from build123d import *

# Parameters (mm, degrees)
F0_W     = 266.7
F0_H     = 152.4
F1_DEPTH = 50.8
F2_R     = 19.05
F3_DEPTH = 50.801
F4_R     = 19.05
F5_DEPTH = 50.801
F6_R     = 6.35


with BuildPart() as f1:
    # F0 (on Front) → F1 (new body)
    with BuildSketch(Plane.XZ):
        Rectangle(F0_W, F0_H)
    extrude(amount=F1_DEPTH)

    # F2 (on Front) → F3 (cut, through all)
    with BuildSketch(Plane.XZ):
        Circle(F2_R)
    extrude(amount=F3_DEPTH, mode=Mode.SUBTRACT)

    # F4 (on Front) → F5 (cut, through all)
    with BuildSketch(Plane.XZ):
        with Locations((-63.5, 0)):
            Circle(F4_R)
        with BuildLine():
            ThreePointArc((82.55, 0), (63.5, 19.05), (44.45, 0))
            ThreePointArc((44.45, 0), (63.5, -19.05), (82.55, 0))
        make_face()
    extrude(amount=F5_DEPTH, mode=Mode.SUBTRACT)

    # F6
    f6_edges = [f1.edges().sort_by_distance(p)[0] for p in [
        (-133.35, -50.8, 0),
        (0, -50.8, -76.2),
        (0, -50.8, 76.2),
        (133.35, -50.8, 0),
        (-133.35, -25.4, -76.2),
        (0, 0, -76.2),
        (-133.35, 0, 0),
        (133.35, -25.4, -76.2),
        (133.35, 0, 0),
        (0, 0, 76.2),
    ]]
    fillet(f6_edges, radius=F6_R)


solid = f1.part
Input: part model. Units: mm. Frame: model coordinates. Coordinates: 2 decimals unless noted, no trailing zeros. Loops run counter-clockwise (first coordinate to the right, second up) from the corner with the lowest first, then second, coordinate; pieces in that order, holes last. Notation, with made-up numbers: (-10, 48) -> (41, 48) arc R4 ccw to (41, 55) -> close; hole circle Ø2 at (-28.5, 51.5). An arc over 180 degrees is marked (long way). Write item = value, one per line. Start each with the question number.
Item 1: Cut plane C-C, the plane y = -11. Return loops of the section in (x, z), plus the area to 3 significant figures.
Item 2: Cut plane A-A, the plane x = 63.5. Return loops of the section in (y, z).
Item 3: Material intervals for line 1 (X direction, y = -3.5, z = 3); line 2 (X direction, y = -46.5, z = 1); line 3 (Z direction, x = 0, y = -32), sorted ascending.
Item 4: Cut plane D-D, the plane x = -53.5. Return loops of the section in (y, z), plus the area to 3 significant figures.
Item 5: Mould query, pull axis X, two halves, no side actions, for faces 1 (the face through (82.53, -25.04, -0.84)), 2 (the face through (-2, -25, 76.2)), 3 (the face through (131.44, -25.67, -74.39)). Classes: pulls with the +X half, pulls with the -X half, needs draft (parallel to the pull), parting line crosses it, or undercut.
Item 6: Cut plane B-B, the plane z = 0. Return loops of the section in (x, y), plus the area to 3 significant figures.
Ans:
q1.outline = (-133.35, -69.85) arc R6.35 ccw to (-127, -76.2) -> (127, -76.2) arc R6.35 ccw to (133.35, -69.85) -> (133.35, 76.2) -> (-133.35, 76.2) -> close; hole circle Ø38.1 at (-63.5, 0); hole circle Ø38.1 at (0, 0); hole circle Ø38.1 at (63.5, 0)
q1.area = 37,200 mm²
q2.outline = (-50.8, -69.85) arc R6.35 ccw to (-44.45, -76.2) -> (-6.35, -76.2) arc R6.35 ccw to (0, -69.85) -> (0, -19.05) -> (-50.8, -19.05) -> close; (-50.8, 19.05) -> (0, 19.05) -> (0, 69.85) arc R6.35 ccw to (-6.35, 76.2) -> (-44.45, 76.2) arc R6.35 ccw to (-50.8, 69.85) -> close
q3.line_1 = -132.67 to -82.31, -44.69 to -18.81, 18.81 to 44.69, 82.31 to 132.67
q3.line_2 = -133.01 to -82.52, -44.48 to -19.02, 19.02 to 44.48, 82.52 to 133.01
q3.line_3 = -76.2 to -19.05, 19.05 to 76.2
q4.outline = (-50.8, -69.85) arc R6.35 ccw to (-44.45, -76.2) -> (-6.35, -76.2) arc R6.35 ccw to (0, -69.85) -> (0, -16.21) -> (-50.8, -16.21) -> close; (-50.8, 16.21) -> (0, 16.21) -> (0, 69.85) arc R6.35 ccw to (-6.35, 76.2) -> (-44.45, 76.2) arc R6.35 ccw to (-50.8, 69.85) -> close
q4.area = 6,060 mm²
q5.face_1 = undercut
q5.face_2 = needs draft
q5.face_3 = pulls with the +X half
q6.outline = (-133.35, -44.45) arc R6.35 ccw to (-127, -50.8) -> (-82.55, -50.8) -> (-82.55, 0) -> (-127, 0) arc R6.35 ccw to (-133.35, -6.35) -> close; (-44.45, -50.8) -> (-19.05, -50.8) -> (-19.05, 0) -> (-44.45, 0) -> close; (19.05, -50.8) -> (44.45, -50.8) -> (44.45, 0) -> (19.05, 0) -> close; (82.55, -50.8) -> (127, -50.8) arc R6.35 ccw to (133.35, -44.45) -> (133.35, -6.35) arc R6.35 ccw to (127, 0) -> (82.55, 0) -> close
q6.area = 7,710 mm²
